```python
from build123d import *

# Parameters (mm, degrees)
SKETCH2_R           = 18.85
BOSS_EXTRUDE1_DEPTH = 2
BOSS_EXTRUDE2_START = -1
SKETCH3_R           = 30
SKETCH3_R_2         = 18.85
BOSS_EXTRUDE2_DEPTH = 1
SKETCH4_R           = 2.9
BOSS_EXTRUDE3_DEPTH = 2
SKETCH6_R           = 5
BOSS_EXTRUDE4_DEPTH = 1
BOSS_EXTRUDE5_DEPTH = 2
SKETCH13_R          = 3
BOSS_EXTRUDE6_DEPTH = 2


with BuildPart() as part:
    # Sketch2 → Boss-Extrude1 (new body)
    with BuildSketch(Plane.XY.offset(10)):
        Circle(SKETCH2_R)
        with BuildLine():
            ThreePointArc((-1.294063412, 15.999741695), (-0.003455665, 17.290865413), (1.287668054, 16.000257666))
            Line((1.287668054, 16.000257666), (1.290071734, 3.973134201))
            Line((1.290071734, 3.973134201), (8.357492916, 13.704694326))
            ThreePointArc((8.357492916, 13.704694326), (10.160519997, 13.990635156), (10.446460828, 12.187608075))
            Line((10.446460828, 12.187608075), (3.379039645, 2.45604795))
            Line((3.379039645, 2.45604795), (14.816771011, 6.17491953))
            ThreePointArc((14.816771011, 6.17491953), (16.443522365, 5.346457793), (15.615060628, 3.71970644))
            Line((15.615060628, 3.71970644), (4.177329262, 0.00083486))
            Line((4.177329262, 0.00083486), (15.616546184, -3.713464648))
            ThreePointArc((15.616546184, -3.713464648), (16.445658083, -5.339884727), (14.819238004, -6.168996626))
            Line((14.819238004, -6.168996626), (3.380021082, -2.454697118))
            Line((3.380021082, -2.454697118), (10.451331501, -12.183431547))
            ThreePointArc((10.451331501, -12.183431547), (10.166111381, -13.986572778), (8.362970151, -13.701352658))
            Line((8.362970151, -13.701352658), (1.291659732, -3.972618229))
            Line((1.291659732, -3.972618229), (1.294063412, -15.999741695))
            ThreePointArc((1.294063412, -15.999741695), (0.003455665, -17.290865413), (-1.287668054, -16.000257666))
            Line((-1.287668054, -16.000257666), (-1.290071734, -3.973134201))
            Line((-1.290071734, -3.973134201), (-8.357492916, -13.704694326))
            ThreePointArc((-8.357492916, -13.704694326), (-10.160519997, -13.990635156), (-10.446460828, -12.187608075))
            Line((-10.446460828, -12.187608075), (-3.379039645, -2.45604795))
            Line((-3.379039645, -2.45604795), (-14.816771011, -6.17491953))
            ThreePointArc((-14.816771011, -6.17491953), (-16.443522365, -5.346457793), (-15.615060628, -3.71970644))
            Line((-15.615060628, -3.71970644), (-4.177329262, -0.00083486))
            Line((-4.177329262, -0.00083486), (-15.616546184, 3.713464648))
            ThreePointArc((-15.616546184, 3.713464648), (-16.445658083, 5.339884727), (-14.819238004, 6.168996626))
            Line((-14.819238004, 6.168996626), (-3.380021082, 2.454697118))
            Line((-3.380021082, 2.454697118), (-10.451331501, 12.183431547))
            ThreePointArc((-10.451331501, 12.183431547), (-10.166111381, 13.986572778), (-8.362970151, 13.701352658))
            Line((-8.362970151, 13.701352658), (-1.291659732, 3.972618229))
            Line((-1.291659732, 3.972618229), (-1.294063412, 15.999741695))
        make_face(mode=Mode.SUBTRACT)
    extrude(amount=BOSS_EXTRUDE1_DEPTH)

    # Sketch3 → Boss-Extrude2 (add)
    with BuildSketch(Plane.XY.offset(12).offset(BOSS_EXTRUDE2_START)):
        Circle(SKETCH3_R)
        Circle(SKETCH3_R_2, mode=Mode.SUBTRACT)
    extrude(amount=BOSS_EXTRUDE2_DEPTH)

    # Sketch4 → Boss-Extrude3 (add)
    with BuildSketch(Plane.XY.offset(12)):
        with Locations((0, 25)):
            Circle(SKETCH4_R)
        with Locations((21.650635095, -12.5)):
            Circle(SKETCH4_R)
        with Locations((-21.650635095, -12.5)):
            Circle(SKETCH4_R)
    extrude(amount=BOSS_EXTRUDE3_DEPTH)

    # Sketch6 → Boss-Extrude4 (add)
    with BuildSketch(Plane(origin=(0, 0, 11), x_dir=(-1, 0, 0), z_dir=(0, 0, -1))):
        with Locations((0, 30)):
            Circle(SKETCH6_R)
        with Locations((25.980762114, -15)):
            Circle(SKETCH6_R)
        with Locations((-25.980762114, -15)):
            Circle(SKETCH6_R)
    extrude(amount=-BOSS_EXTRUDE4_DEPTH)

    # Sketch12 → Boss-Extrude5 (add)
    with BuildSketch(Plane(origin=(0, 0, 10), x_dir=(-1, 0, 0), z_dir=(0, 0, -1))):
        with BuildLine():
            Line((-2.213684697, 5.244912811), (-1.382375366, 2.662524807))
            ThreePointArc((-1.382375366, 2.662524807), (-0.919286358, 2.855680758), (-0.43048178, 2.968953593))
            Line((-0.43048178, 2.968953593), (-1.28973897, 5.638159118))
            Line((-1.28973897, 5.638159118), (-1.290071734, 3.973134201))
            Line((-1.290071734, 3.973134201), (-2.213684697, 5.244912811))
        make_face()
        with BuildLine():
            Line((1.291973859, 5.544394816), (0.446627652, 2.96656767))
            ThreePointArc((0.446627652, 2.96656767), (0.934808749, 2.850637228), (1.396840061, 2.654964754))
            Line((1.396840061, 2.654964754), (2.270606035, 5.31945609))
            Line((2.270606035, 5.31945609), (1.291659732, 3.972618229))
            Line((1.291659732, 3.972618229), (1.291973859, 5.544394816))
        make_face()
        with BuildLine():
            ThreePointArc((2.105034087, 2.137482513), (2.431838686, 1.756747166), (2.690616475, 1.326869617))
            Line((2.690616475, 1.326869617), (4.963656709, 2.968901637))
            Line((4.963656709, 2.968901637), (3.380021082, 2.454697118))
            Line((3.380021082, 2.454697118), (4.304142315, 3.726106449))
            Line((4.304142315, 3.726106449), (2.105034087, 2.137482513))
        make_face()
        with BuildLine():
            ThreePointArc((3, 0), (2.989147583, -0.254944562), (2.956668847, -0.508044614))
            Line((2.956668847, -0.508044614), (5.76075923, -0.515672332))
            Line((5.76075923, -0.515672332), (4.177329262, -0.00083486))
            Line((4.177329262, -0.00083486), (5.672274698, 0.484572064))
            Line((5.672274698, 0.484572064), (2.959389048, 0.491951686))
            ThreePointArc((2.959389048, 0.491951686), (2.989830024, 0.246812536), (3, 0))
        make_face()
        with BuildLine():
            ThreePointArc((2.683357979, -1.341487964), (2.422245321, -1.7699513), (2.093374212, -2.148903071))
            Line((2.093374212, -2.148903071), (4.357447525, -3.803276998))
            Line((4.357447525, -3.803276998), (3.379039645, -2.45604795))
            Line((3.379039645, -2.45604795), (4.87379094, -2.94205238))
            Line((4.87379094, -2.94205238), (2.683357979, -1.341487964))
        make_face()
        with BuildLine():
            ThreePointArc((1.382375366, -2.662524807), (0.919286358, -2.855680758), (0.43048178, -2.968953593))
            Line((0.43048178, -2.968953593), (1.28973897, -5.638159118))
            Line((1.28973897, -5.638159118), (1.290071734, -3.973134201))
            Line((1.290071734, -3.973134201), (2.213684697, -5.244912811))
            Line((2.213684697, -5.244912811), (1.382375366, -2.662524807))
        make_face()
        with BuildLine():
            Line((-1.396840061, -2.654964754), (-2.270606035, -5.31945609))
            Line((-2.270606035, -5.31945609), (-1.291659732, -3.972618229))
            Line((-1.291659732, -3.972618229), (-1.291973859, -5.544394816))
            Line((-1.291973859, -5.544394816), (-0.446627652, -2.96656767))
            ThreePointArc((-0.446627652, -2.96656767), (-0.934808749, -2.850637228), (-1.396840061, -2.654964754))
        make_face()
        with BuildLine():
            Line((-4.304142315, -3.726106449), (-2.105034087, -2.137482513))
            ThreePointArc((-2.105034087, -2.137482513), (-2.431838686, -1.756747166), (-2.690616475, -1.326869617))
            Line((-2.690616475, -1.326869617), (-4.963656709, -2.968901637))
            Line((-4.963656709, -2.968901637), (-3.380021082, -2.454697118))
            Line((-3.380021082, -2.454697118), (-4.304142315, -3.726106449))
        make_face()
        with BuildLine():
            Line((-5.672274698, -0.484572064), (-2.959389048, -0.491951686))
            ThreePointArc((-2.959389048, -0.491951686), (-2.999988901, 0.008160604), (-2.956668847, 0.508044614))
            Line((-2.956668847, 0.508044614), (-5.76075923, 0.515672332))
            Line((-5.76075923, 0.515672332), (-4.177329262, 0.00083486))
            Line((-4.177329262, 0.00083486), (-5.672274698, -0.484572064))
        make_face()
        with BuildLine():
            Line((-4.87379094, 2.94205238), (-2.683357979, 1.341487964))
            ThreePointArc((-2.683357979, 1.341487964), (-2.422245321, 1.7699513), (-2.093374212, 2.148903071))
            Line((-2.093374212, 2.148903071), (-4.357447525, 3.803276998))
            Line((-4.357447525, 3.803276998), (-3.379039645, 2.45604795))
            Line((-3.379039645, 2.45604795), (-4.87379094, 2.94205238))
        make_face()
    extrude(amount=-BOSS_EXTRUDE5_DEPTH)

    # Sketch13 → Boss-Extrude6 (add)
    with BuildSketch(Plane(origin=(0, 0, 10), x_dir=(-1, 0, 0), z_dir=(0, 0, -1))):
        Circle(SKETCH13_R)
    extrude(amount=-BOSS_EXTRUDE6_DEPTH)


solid = part.part
```
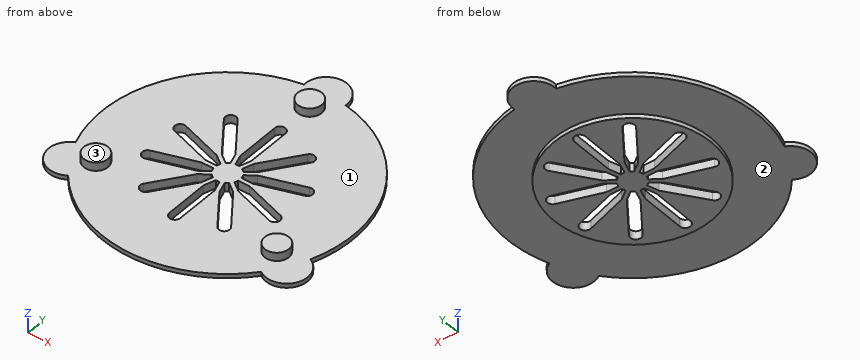
Build history of the part. All positions in model axes, mm. Face numbers are marked on the shaded views. A direction names the side the tool comes from. Round coordinates to 2 decimals unless told otherwise and drop trailing zeros. Loops run counter-clockwise (first coordinate to the right, second up) from the corner with the lowest first, then second, coordinate; pieces in that order, holes last.
Item 1: Saw through at A-A (y = 7.5). List the corners of the cut face in (x, z).
Item 2: Drill centre lines: line 1 along Y through (x, z) = (14, 11.4); line 2 along X through (y, z) = (-12, 13.85); line 3 along Z through (x, y) = (-27, -11). Where is each one in solid material? Low to high.
Item 3: Saw through at C-C (x = -22). List the corners of the cut face in (y, z).
Item 4: Saw through at D-D (y = 21). List the corners of the cut face in (x, z).
Item 5: Saw through at B-B (z = 13). List the corners of the cut face in (x, y), then the cut area to 3 significant figures.
Item 6: Which spindle directions (+Z, -Z, +X, -X, +Y, -Y) get a long thin tool onto all of the face, cutting with end or side? Do the marked faces 1, 2 and 3. Say none if no direction does.
Item 7: Pin check, flat tips, straight feed: P1, Ø1, axis at y = 9.5, z = 11, coming from the +X side; P2, Ø1.6, axis at y = -9.5, z = 11, coming from the +X side; P3, Ø1, axis at y = 9, z = 11, coming from the -X side. Stop position of each tip, or through.
Worked answers:
1. outline: (-29.05, 11) - (-17.29, 11) - (-17.29, 10) - (-7.05, 10) - (-7.05, 12) - (-29.05, 12) - close; (-3.86, 10) - (-1.29, 10) - (-1.29, 12) - (-3.86, 12) - close; (1.29, 10) - (3.85, 10) - (3.85, 12) - (1.29, 12) - close; (7.04, 10) - (17.29, 10) - (17.29, 11) - (29.05, 11) - (29.05, 12) - (7.04, 12) - close
2. line 1: y = -26.53 to -5.9, -3.19 to 3.19, 5.91 to 26.53
2. line 2: x = -24.51 to -18.79, 18.79 to 24.51
2. line 3: z = 11 to 12
3. outline: (-20.4, 11) - (20.4, 11) - (20.4, 12) - (-9.62, 12) - (-9.62, 14) - (-15.38, 14) - (-15.38, 12) - (-20.4, 12) - close
4. outline: (-21.42, 11) - (21.42, 11) - (21.42, 12) - (-21.42, 12) - close
5. outline: circle Ø5.8 at (-21.65, -12.5); circle Ø5.8 at (0, 25); circle Ø5.8 at (21.65, -12.5)
5. area: 79.3 mm2
6. face 1: +Z
6. face 2: -Z
6. face 3: +Z, +X, -X, +Y, -Y
7. P1: stops at x = 28.62
7. P2: stops at x = 28.71
7. P3: stops at x = -28.77
